Read the model definition and answer for the solid it produces. Units are mm, in the model's axes. A direction names the side the tool comes from. Give positions to 0.01 mm unless a question says otherwise; leave off trailing zeros. Order: outer loops, then holes, each group sorted by start corner. A loop starts at its lowest first (then second) coordinate and runs counter-clockwise, first axis right, second up. Notation, with made-up numbers: (-4, 37) - (46, 37) arc R22 cw to (46, 45) - close; hole circle Ø4 at (42.25, 59). An arc over 180 degrees is marked (long way). Use a Markdown table: item, result. Add a question column.
1. Consider L1, parallel to X at y = 11, z = 28.5; L2, parallel to Y at x = -10.5, z = -13.5; L3, parallel to X at y = 35.5, z = -15. Determine where each line is inside the solid, lowest interval first.
2. A cutting plane is placed at C-C on z = -4. Determine the outline of the cut face in (x, y), and give its area (3 significant figures).
3. Flat-ended cylindrical pins translate along their axes: P1, Ø0.8, axis at x = 0.5, z = 25, coming from the -Y side; P2, Ø1.5, axis at y = 16.5, z = -1, coming from the -X side; P3, Ø3, axis at x = -21.5, z = -3.5, coming from the +Y side. Find the tip coordinate at first contact, or state that the pin passes through.
4. For a pull along Z with two mould halves and no side action, classify faces 1 (the flat face through (-20.32, 8, 1)), 2 (the cylindrical face through (-9.15, -1.25, -26.11)), 3 (the cylindrical face through (1.29, 46.35, 36.29)), 4 (the cylindrical face through (-21.57, 10.79, -36.29)) as released by +Z, released by -Z, zero draft, split by the parting line, or undercut.
5. A cutting plane is placed at A-A on x = -10.16. Determine the outline of the cut face in (y, z).
6. A cutting plane is placed at D-D on y = 34.5. Determine the outline of the cut face in (x, z).
7. Which of the six approach directions +Z, -Z, +X, -X, +Y, -Y give full straight-line access (tool end or side, diameter ignored) to faces 5 (the cylindrical face through (1.29, 35.63, 31.75)), 6 (the flat face through (-10, -2.54, 1)), 7 (the flat face through (0, 25, 1)), 8 (the cylindrical face through (-21.57, 10.79, 36.29))?
8. A cutting plane is placed at B-B on z = 25. Determine the outline of the cut face in (x, y) (3 decimals), and give its area (3 significant figures).
```python
from build123d import *

# Parameters (mm, degrees)
BOSS_EXTRUDE1_DEPTH      = 38.1
CUT_EXTRUDE1_DEPTH       = 66.598911576
CUT_EXTRUDE1_DEPTH_BACK  = 66.598911576
FILLET1_R                = 6.35
FILLET2_R                = 2.54
FILLET3_R                = 5.08
SCHIZZO1_R               = 1.5
TAGLIO_ESTRUSIONE1_DEPTH = 10


with BuildPart() as part:
    # Sketch1 → Boss-Extrude1 (new, symmetric)
    with BuildSketch(Plane.XY):
        Polygon((0, 0), (0, 48.26), (2.54, 48.26), (2.54, -2.54), (-22.86, -2.54), (-22.86, 0), (-22.86, 12.7), (-20.32, 12.7), (-20.32, 0), align=None)
    extrude(amount=BOSS_EXTRUDE1_DEPTH, both=True)

    # Sketch2 → Cut-Extrude1 (cut, two sides: drawn at the far end of the back side and taken through both)
    with BuildSketch(Plane.ZY.offset(-CUT_EXTRUDE1_DEPTH_BACK)):
        with BuildLine():
            Line((-28.575, 38.735), (-19.05, 38.735))
            ThreePointArc((-19.05, 38.735), (-15.875, 35.56), (-19.05, 32.385))
            Line((-19.05, 32.385), (-28.575, 32.385))
            ThreePointArc((-28.575, 32.385), (-31.75, 35.56), (-28.575, 38.735))
        make_face()
        with BuildLine():
            Line((19.05, 38.735), (28.575, 38.735))
            ThreePointArc((28.575, 38.735), (31.75, 35.56), (28.575, 32.385))
            Line((28.575, 32.385), (19.05, 32.385))
            ThreePointArc((19.05, 32.385), (15.875, 35.56), (19.05, 38.735))
        make_face()
    extrude(amount=CUT_EXTRUDE1_DEPTH + CUT_EXTRUDE1_DEPTH_BACK, mode=Mode.SUBTRACT)

    # Fillet1
    fillet1_edges = [part.edges().sort_by_distance(p)[0] for p in [
        (-21.59, 12.7, 38.1),
        (-21.59, 12.7, -38.1),
        (1.27, 48.26, 38.1),
        (1.27, 48.26, -38.1),
    ]]
    fillet(fillet1_edges, radius=FILLET1_R)

    # Fillet2
    fillet2_edges = [part.edges().sort_by_distance(p)[0] for p in [
        (0, 0, 0),
        (-20.32, 0, 0),
    ]]
    fillet(fillet2_edges, radius=FILLET2_R)

    # Fillet3
    fillet3_edges = [part.edges().sort_by_distance(p)[0] for p in [
        (2.54, -2.54, 0),
        (-22.86, -2.54, 0),
    ]]
    fillet(fillet3_edges, radius=FILLET3_R)

    # Schizzo1 → Taglio-Estrusione1 (cut)
    with BuildSketch(Plane(origin=(0, 0, 0), x_dir=(1, 0, 0), z_dir=(0, 1, 0))):
        with Locations(Location((-10.16, 25, 0), (0, 0, 270))):
            Circle(SCHIZZO1_R)
        with Locations(Location((-10.16, -25, 0), (0, 0, 180))):
            Circle(SCHIZZO1_R)
    extrude(amount=-TAGLIO_ESTRUSIONE1_DEPTH, mode=Mode.SUBTRACT)


solid = part.part
```
Output values:
| question | item | result |
|---|---|---|
| 1 | L1 | -22.86 to -20.32, 0 to 2.54 |
| 1 | L2 | -2.54 to 0 |
| 1 | L3 | 0 to 2.54 |
| 2 | outline | (-22.86, 2.54) arc R5.08 ccw to (-17.78, -2.54) - (-2.54, -2.54) arc R5.08 ccw to (2.54, 2.54) - (2.54, 48.26) - (0, 48.26) - (0, 2.54) arc R2.54 cw to (-2.54, 0) - (-17.78, 0) arc R2.54 cw to (-20.32, 2.54) - (-20.32, 12.7) - (-22.86, 12.7) - close |
| 2 | area | 211 mm² |
| 3 | P1 | y = -1.8 |
| 3 | P2 | x = 0 |
| 3 | P3 | y = 12.7 |
| 4 | face 1 | zero draft |
| 4 | face 2 | undercut |
| 4 | face 3 | released by +Z |
| 4 | face 4 | released by -Z |
| 5 | outline | (-2.54, -38.1) - (0, -38.1) - (0, -26.5) - (-2.54, -26.5) - close; (-2.54, -23.5) - (0, -23.5) - (0, 23.5) - (-2.54, 23.5) - close; (-2.54, 26.5) - (0, 26.5) - (0, 38.1) - (-2.54, 38.1) - close |
| 6 | outline | (0, -38.1) - (2.54, -38.1) - (2.54, -31.57) - (0, -31.57) - close; (0, -16.06) - (2.54, -16.06) - (2.54, 16.06) - (0, 16.06) - close; (0, 31.57) - (2.54, 31.57) - (2.54, 38.1) - (0, 38.1) - close |
| 7 | face 5 | +X, -X |
| 7 | face 6 | +Z, -Z, +X, -X, -Y |
| 7 | face 7 | +Z, -Z, +Y |
| 7 | face 8 | +Z, -X, +Y |
| 8 | outline | (-22.86, 2.54) arc R5.08 ccw to (-17.78, -2.54) - (-11.66, -2.54) - (-11.66, 0) - (-17.78, 0) arc R2.54 cw to (-20.32, 2.54) - (-20.32, 12.7) - (-22.86, 12.7) - close; (-8.66, -2.54) - (-2.54, -2.54) arc R5.08 ccw to (2.54, 2.54) - (2.54, 32.385) - (0, 32.385) - (0, 2.54) arc R2.54 cw to (-2.54, 0) - (-8.66, 0) - close; (0, 38.735) - (2.54, 38.735) - (2.54, 48.26) - (0, 48.26) - close |
| 8 | area | 187 mm² |
